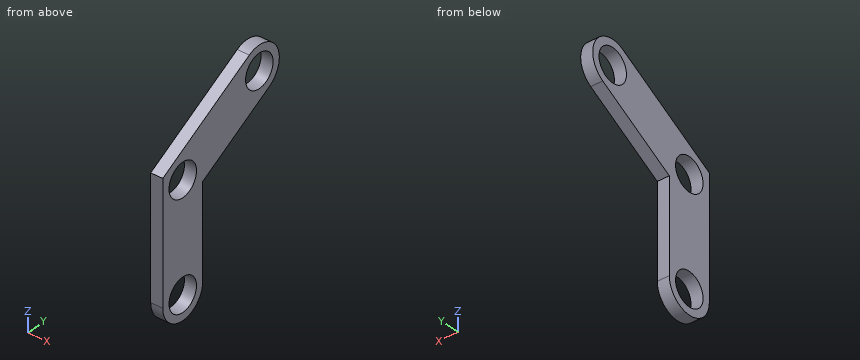
```python
from build123d import *

# Parameters (mm, degrees)
SKETCH1_R           = 2.75
BOSS_EXTRUDE1_DEPTH = 2


with BuildPart() as part:
    # Sketch1 → Boss-Extrude1 (new body)
    with BuildSketch(Plane(origin=(0, 0, 0), x_dir=(0, 0, -1), z_dir=(1, 0, 0))):
        with BuildLine():
            Line((0, 0), (-10, 17.320508076))
            ThreePointArc((-10, 17.320508076), (-8.535898385, 22.784609691), (-3.07179677, 21.320508076))
            Line((-3.07179677, 21.320508076), (4.618802154, 8))
            Line((4.618802154, 8), (20, 8))
            ThreePointArc((20, 8), (24, 4), (20, 0))
            Line((20, 0), (0, 0))
        make_face()
        with Locations((-6.535898385, 19.320508076)):
            Circle(SKETCH1_R, mode=Mode.SUBTRACT)
        with Locations((20, 4)):
            Circle(SKETCH1_R, mode=Mode.SUBTRACT)
        with Locations((2.309401077, 4)):
            Circle(SKETCH1_R, mode=Mode.SUBTRACT)
    extrude(amount=BOSS_EXTRUDE1_DEPTH)


solid = part.part
```
Model file for the job. Use its own axes, mm. Coordinates: 2 decimals unless noted, no trailing zeros. Write each loop counter-clockwise with the first axis right and the second up, starting at its lowest first coordinate (ties: lowest second). Pieces come first, ordered by that corner, then holes. Notation, with made-up numbers: (55, 65) - (113, 65) arc R24 ccw to (113, 101) - close; hole circle Ø11 at (70.5, 49.5). An arc over 180 degrees is marked (long way). One line per item, written item: value. Start each with the question number.
1. Probe line 1 (Z direction, x = 1.1, y = 2.5); line 2 (Z direction, x = 1.3, y = 3.5); line 3 (Y direction, x = 1.25, z = -9.5). List the from-to ranges inside material, lowest first. Write a range as from..to.
2. Slice it at B-B (x = 0.3). Write the cut outline in (y, z), plus the area to 3 significant figures.
3. Flat gauge pins, fed straight in: pin 1 (0.6 mm diameter, centred on x = 1, z = -15.5, fed in from +Y); pin 2 (1 mm diameter, centred on x = 0.5, y = 6, fed in from +Z). Where does each tip first touch, or does it go through?
4. Slice it at A-A (z = -21). Write the cut outline in (x, y).
5. Slice it at D-D (y = 4). Write the cut outline in (x, z).
6. Slice it at C-C (y = 20.5). Write the cut outline in (x, z), plus the area to 3 significant figures.
Answers below:
1. line 1: z = -23.71..-22.3, -17.7..-4.61, 0..1.44
1. line 2: z = -23.97..-22.7, -17.3..-5.01, 0.39..2.02
1. line 3: y = 0..8
2. outline: (0, -20) arc R4 ccw to (8, -20) - (8, -4.62) - (21.32, 3.07) arc R4 ccw to (17.32, 10) - (0, 0) - close; hole circle Ø5.5 at (4, -20); hole circle Ø5.5 at (4, -2.31); hole circle Ø5.5 at (19.32, 6.54)
2. area: 262 mm^2
3. pin 1: stops at y = 8
3. pin 2: stops at z = 3.75
4. outline: (0, 0.13) - (2, 0.13) - (2, 1.44) - (0, 1.44) - close; (0, 6.56) - (2, 6.56) - (2, 7.87) - (0, 7.87) - close
5. outline: (0, -24) - (2, -24) - (2, -22.75) - (0, -22.75) - close; (0, -17.25) - (2, -17.25) - (2, -5.06) - (0, -5.06) - close; (0, 0.44) - (2, 0.44) - (2, 2.31) - (0, 2.31) - close
6. outline: (0, 2.6) - (2, 2.6) - (2, 4.05) - (0, 4.05) - close; (0, 9.02) - (2, 9.02) - (2, 10.36) - (0, 10.36) - close
6. area: 5.58 mm^2
